For this review, take the finished solid that the model builds, in its own axes (mm). Face numbers are marked on the shaded views. A direction names the side the tool comes from. Round coordinates to 2 decimals unless told otherwise and drop trailing zeros. Write each loop counter-clockwise with the first axis right and the second up, starting at its lowest first coordinate (ties: lowest second). Pieces come first, ordered by that corner, then holes. Notation, with made-up numbers: (48.5, 14.5) -> (54.5, 14.5) arc R13 ccw to (54.5, 29.5) -> close; hole circle Ø10 at (60, -25). An arc over 180 degrees is marked (long way). Answer in a Markdown table with one row per item.
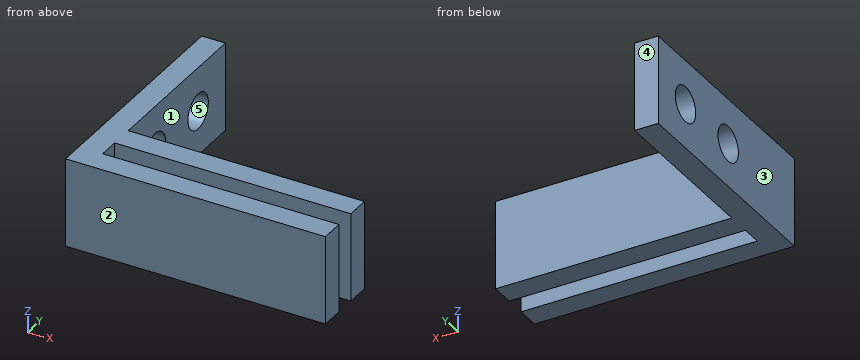
from build123d import *

# Parameters (mm, degrees)
SKETCH1_W           = 7.5
SKETCH1_H           = 20
BOSS_EXTRUDE2_DEPTH = 2
SKETCH2_W           = 7.5
SKETCH2_H           = 1.98347932
BOSS_EXTRUDE3_DEPTH = 20
SKETCH3_W           = 7.5
SKETCH3_H           = 2
BOSS_EXTRUDE4_DEPTH = 20
SKETCH5_R           = 1.5
CUT_EXTRUDE1_DEPTH  = 20


with BuildPart() as part:
    # Sketch1 → Boss-Extrude2 (new body)
    with BuildSketch(Plane(origin=(0, 0, 0), x_dir=(0, 0, -1), z_dir=(1, 0, 0))):
        with Locations((3.009581882, -0.975609756)):
            Rectangle(SKETCH1_W, SKETCH1_H)
    extrude(amount=BOSS_EXTRUDE2_DEPTH)

    # Sketch2 → Boss-Extrude3 (add)
    with BuildSketch(Plane(origin=(2, 0, 0), x_dir=(0, 0, -1), z_dir=(1, 0, 0))):
        with Locations((3.009581882, -9.983870096)):
            Rectangle(SKETCH2_W, SKETCH2_H)
    extrude(amount=BOSS_EXTRUDE3_DEPTH)

    # Sketch3 → Boss-Extrude4 (add)
    with BuildSketch(Plane(origin=(2, 0, 0), x_dir=(0, 0, -1), z_dir=(1, 0, 0))):
        with Locations((3.009581882, -6.242130436)):
            Rectangle(SKETCH3_W, SKETCH3_H)
    extrude(amount=BOSS_EXTRUDE4_DEPTH)

    # Sketch5 → Cut-Extrude1 (cut)
    with BuildSketch(Plane(origin=(2, 0, 0), x_dir=(0, 0, -1), z_dir=(1, 0, 0))):
        with Locations((3.009581882, 5.024390244)):
            Circle(SKETCH5_R)
        with Locations((3.096458319, -1.242130436)):
            Circle(SKETCH5_R)
    extrude(amount=-CUT_EXTRUDE1_DEPTH, mode=Mode.SUBTRACT)


solid = part.part
1) Consider section B-B on z = -6. State the section outline as (x, y) points.
Solved:
| item | result |
|---|---|
| outline | (0, -10.98) -> (22, -10.98) -> (22, -8.99) -> (2, -8.99) -> (2, -7.24) -> (22, -7.24) -> (22, -5.24) -> (2, -5.24) -> (2, 9.02) -> (0, 9.02) -> close |
2) Consider section C-C on z = -3.5. State the section outline as (x, y) points, then the cut area to 3 significant figures.
Solved:
| item | result |
|---|---|
| outline | (0, -10.98) -> (22, -10.98) -> (22, -8.99) -> (2, -8.99) -> (2, -7.24) -> (22, -7.24) -> (22, -5.24) -> (2, -5.24) -> (2, -2.69) -> (0, -2.69) -> close; (0, 0.2) -> (2, 0.2) -> (2, 3.61) -> (0, 3.61) -> close; (0, 6.44) -> (2, 6.44) -> (2, 9.02) -> (0, 9.02) -> close |
| area | 108 mm² |
3) Clearance check with flat-ended pins moving along their axes: pin 1 Ø12 at (x, y) = (7.5, 6.5) entering from -Z; pin 2 Ø4 at (x, z) = (10, -3) entering from +Y; pin 3 Ø3.5 at (y, z) = (-1.24, -3.1) entering from +X. State where each tip first meets the part, or that it passes through.
Solved:
| item | result |
|---|---|
| pin 1 | z = -6.76 |
| pin 2 | y = -5.24 |
| pin 3 | x = 2 |
4) For line 1 (Y direction, x = 11.25, z = -4.25); line 2 (X direction, y = -8.25, z = -5.5), list the stretches that pass through material, from the lowest coordinate up. Write a range as [from, to].
Solved:
| item | result |
|---|---|
| line 1 | [-10.98, -8.99], [-7.24, -5.24] |
| line 2 | [0, 2] |
5) Consider section D-D on y = -4.5. State the section outline as (x, z) points.
Solved:
| item | result |
|---|---|
| outline | (0, -6.76) -> (2, -6.76) -> (2, 0.74) -> (0, 0.74) -> close |
6) Mouldability with a two-part tool opening along Y and no side actions: class the marked faces 3, 4 and 5 as pulls with the +Y half, pulls with the -Y half, needs draft (parallel to the pull), parting line crosses it, or undercut.
Solved:
| item | result |
|---|---|
| face 3 | needs draft |
| face 4 | pulls with the +Y half |
| face 5 | undercut |
7) For the marked faces 1 and 2, list the 3-axis set-ups (+Z, -Z, +X, -X, +Y, -Y) from which the entire face can be reached by the end or side of a thin tool; tool diameter is ignored.
Solved:
| item | result |
|---|---|
| face 1 | +Z, -Z, +X, +Y |
| face 2 | +Z, -Z, +X, -X, -Y |
8) Consider section A-A on x = 17.75. State the section outline as (y, z) points.
Solved:
| item | result |
|---|---|
| outline | (-10.98, -6.76) -> (-8.99, -6.76) -> (-8.99, 0.74) -> (-10.98, 0.74) -> close; (-7.24, -6.76) -> (-5.24, -6.76) -> (-5.24, 0.74) -> (-7.24, 0.74) -> close |
